from build123d import *

# Parameters (mm, degrees)
SKETCH1_R           = 31
BOSS_EXTRUDE1_DEPTH = 50
BOSS_EXTRUDE2_DEPTH = 6
SKETCH3_R           = 2.3
CUT_EXTRUDE1_DEPTH  = 4


with BuildPart() as part:
    # Sketch1 → Boss-Extrude1 (new body)
    with BuildSketch(Plane(origin=(0, 0, 0), x_dir=(1, 0, 0), z_dir=(0, 1, 0))):
        with Locations(Location((0, 0, 0), (0, 0, 270))):
            Circle(SKETCH1_R)
        with BuildLine():
            Line((25.902702562, -8.3), (26.950881247, -8.3))
            ThreePointArc((26.950881247, -8.3), (28.2, 0), (26.950881247, 8.3))
            Line((26.950881247, 8.3), (25.902702562, 8.3))
            ThreePointArc((25.902702562, 8.3), (-27.2, 0), (25.902702562, -8.3))
        make_face(mode=Mode.SUBTRACT)
    extrude(amount=-BOSS_EXTRUDE1_DEPTH)

    # Sketch2 → Boss-Extrude2 (add)
    with BuildSketch(Plane(origin=(0, 0, 0), x_dir=(1, 0, 0), z_dir=(0, 1, 0))):
        with BuildLine():
            Line((15.994999219, -22), (-15.994999219, -22))
            ThreePointArc((-15.994999219, -22), (0, -27.2), (15.994999219, -22))
        make_face()
        with BuildLine():
            Line((-15.994999219, 22), (15.994999219, 22))
            ThreePointArc((15.994999219, 22), (0, 27.2), (-15.994999219, 22))
        make_face()
        with BuildLine():
            Line((-22, -15.994999219), (-22, 15.994999219))
            ThreePointArc((-22, 15.994999219), (-27.2, 0), (-22, -15.994999219))
        make_face()
    extrude(amount=-BOSS_EXTRUDE2_DEPTH)

    # Sketch3 → Cut-Extrude1 (cut)
    with BuildSketch(Plane(origin=(0, 0, 0), x_dir=(1, 0, 0), z_dir=(0, 1, 0))):
        with Locations(Location((-25.597034397, 6.858704695, 0), (0, 0, 270))):
            Circle(SKETCH3_R)
        with Locations(Location((-25.597034397, -6.858704695, 0), (0, 0, 270))):
            Circle(SKETCH3_R)
        with Locations(Location((-6.858704695, 25.597034397, 0), (0, 0, 270))):
            Circle(SKETCH3_R)
        with Locations(Location((6.858704695, 25.597034397, 0), (0, 0, 270))):
            Circle(SKETCH3_R)
        with Locations(Location((6.858704695, -25.597034397, 0), (0, 0, 270))):
            Circle(SKETCH3_R)
        with Locations(Location((-6.858704695, -25.597034397, 0), (0, 0, 270))):
            Circle(SKETCH3_R)
    extrude(amount=-CUT_EXTRUDE1_DEPTH, mode=Mode.SUBTRACT)


solid = part.part
Geometry: final body of the model. Coordinates: model frame, mm. A direction names the side the tool comes from. Round coordinates to 2 decimals unless told otherwise and drop trailing zeros. Loops run counter-clockwise (first coordinate to the right, second up) from the corner with the lowest first, then second, coordinate; pieces in that order, holes last. Notation, with made-up numbers: M 42,66.5 L 68,66.5 A27 ccw 68,105.5 Z; hole C 41,20 d5. An arc over 180 degrees is marked long. Put each result on its own line as item: value. Start each with the question number.
(1) Section query B-B (z = 0). Return loops of the section in (x, y).
(2) Contact query for flat-ended pins moving along their axis: pin 1 Ø5 at (x, y) = (-22.5, -15) entering from -Z; pin 2 Ø2 at (x, y) = (-8.5, -34) entering from -Z; pin 3 Ø3 at (x, z) = (-6.86, -25.6) entering from -Y; pin 4 Ø4 at (y, z) = (-17.5, -18) entering from -X. Output: stop coordinate, or through.
(3) Section query A-A (x = 14.5). Return loops of the section in (y, z), then the cut area to 3 significant figures.
(4) Section query D-D (x = 0). Return loops of the section in (y, z).
(5) Material intervals for line 1 along Z through (x, y) = (-0.5, -25.5); line 2 along X through (y, z) = (-40, -3); line 3 along Z through (x, y) = (5.5, -17), sorted ascending. Write a range as [from, to].
(6) Draft query along Z for faces 5 (the face through (28.2, -24.6, 0.1)), 6 (the face through (30.736, -24.65, -4.036)), 7 (the face through (-21, -50, 18)). Return one class per face: +Z half, -Z half, draft (parallel to the pull), parting line (faces both ways), or undercut.
(7) Set-up query: faces 1 (the face through (0, -6, -24)), 2 (the face through (-23, 0, 0)), 3 (the face through (-22, -3, 0)), 4 (the face through (-6.76, -1.97, 23.3)). Return all of +Z, -Z, +X, -X, +Y, -Y with unobstructed straight access to the full face (end or side cutting, diameter ignored); none if empty.
(8) Section query C-C (y = -30.5). Return loops of the section in (x, z), then the cut area to 3 significant figures.
Findings below:
1. outline: M -31,-50 L -27.2,-50 L -27.2,-6 L -22,-6 L -22,0 L -31,0 Z; M 28.2,-50 L 31,-50 L 31,0 L 28.2,0 Z
2. pin 1: stops at z = -23.69
2. pin 2: stops at z = -30.08
2. pin 3: stops at y = -50
2. pin 4: stops at x = -26.55
3. outline: M -50,-27.4 L 0,-27.4 L 0,-22 L -6,-22 L -6,-23.01 L -50,-23.01 Z; M -50,23.01 L -6,23.01 L -6,22 L 0,22 L 0,27.4 L -50,27.4 Z
3. area: 451 mm2
4. outline: M -50,-31 L 0,-31 L 0,-22 L -6,-22 L -6,-27.2 L -50,-27.2 Z; M -50,27.2 L -6,27.2 L -6,22 L 0,22 L 0,31 L -50,31 Z
5. line 1: z = [-31, -27.2], [27.2, 31]
5. line 2: x = [-30.85, -27.03], [28.04, 30.85]
5. line 3: z = [-30.51, -26.64], [26.64, 30.51]
6. face 5: undercut
6. face 6: parting line
6. face 7: draft
7. face 1: -Y
7. face 2: +Z, -Z, +X, -X, +Y
7. face 3: +Y, -Y
7. face 4: +Y
8. outline: C 0,0 d62; hole M 25.9,-8.3 L 26.95,-8.3 A28.2 ccw 26.95,8.3 L 25.9,8.3 A27.2 ccw long Z
8. area: 678 mm2
